Can you work these out from the drawing? Everything is in mm from the part's minimum corner. Give positions to 0.01 mm unless a question says otherwise; leave off trailing zeros. Loops run counter-clockwise (first coordinate to the right, second up) from the corner with the lowest first, then second, coordinate; pieces in that order, holes last. Notation, with made-up numbers: (1, -26) - (48, -26) arc R12 cw to (48, -6) - close; hole circle Ø8 at (23.25, 12). An arc over 180 degrees is marked (long way). Answer in a Markdown table with one row per item. Add a question column.
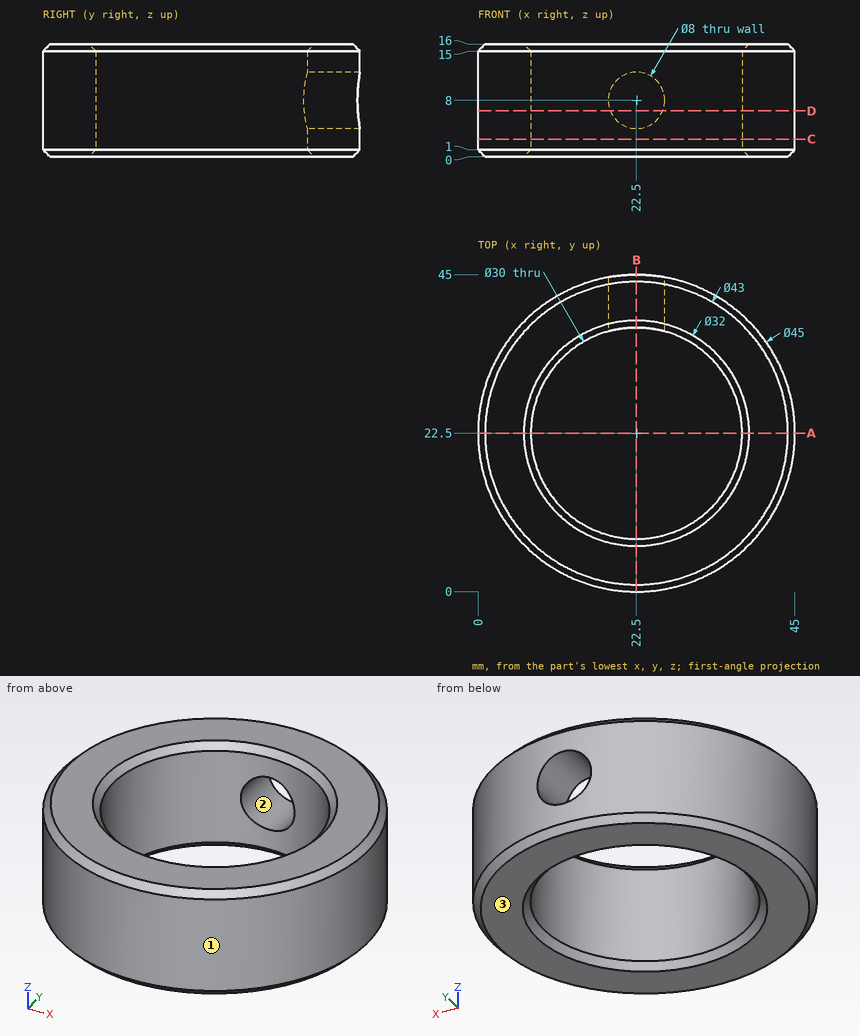
(1) For pin 1 Ø1 at (y, z) = (21, 1.5) entering from -X; pin 2 Ø3 at (x, z) = (31, 4) entering from +Y; pin 3 Ø8 at (y, z) = (31, 4) entering from +X, each with a flat end and sliding along its axis, tell me the tip position at first contact or that it passes through.
(2) I want a section at A-A on y = 22.5. Please give me the cut outline in (x, z).
(3) I want a section at D-D on z = 6.5. Please give me the cut outline in (x, y), then the cut area to 3 significant figures.
(4) We'd pull the mould along X, two halves only. Please class the marked faces 1, 2 and 3: pulls with the +X half, pulls with the -X half, needs draft (parallel to the pull), parting line crosses it, or undercut.
(5) I want a section at B-B on x = 22.5. Please give me the cut outline in (y, z), then the cut area to 3 significant figures.
(6) I want a section at C-C on z = 2.5. Please give me the cut outline in (x, y).
(7) Please list where these lines run through material, in increasing order: line 1 (Z direction, x = 22.5, y = 42); line 2 (Y direction, x = 22.5, z = 4.5); line 3 (X direction, y = 20, z = 2.25).
Reported:
| question | item | result |
|---|---|---|
| 1 | pin 1 | x = 0.02 |
| 1 | pin 2 | y = 43.88 |
| 1 | pin 3 | x = 44.55 |
| 2 | outline | (0, 1) - (1, 0) - (6.5, 0) - (7.5, 1) - (7.5, 15) - (6.5, 16) - (1, 16) - (0, 15) - close; (37.5, 1) - (38.5, 0) - (44, 0) - (45, 1) - (45, 15) - (44, 16) - (38.5, 16) - (37.5, 15) - close |
| 3 | outline | (18.79, 37.03) - (18.79, 44.69) arc R22.5 ccw (long way) to (26.21, 44.69) - (26.21, 37.03) arc R15 cw (long way) to start |
| 3 | area | 828 mm² |
| 4 | face 1 | parting line crosses it |
| 4 | face 2 | undercut |
| 4 | face 3 | needs draft |
| 5 | outline | (0, 1) - (1, 0) - (6.5, 0) - (7.5, 1) - (7.5, 15) - (6.5, 16) - (1, 16) - (0, 15) - close; (37.5, 1) - (38.5, 0) - (44, 0) - (45, 1) - (45, 4) - (37.5, 4) - close; (37.5, 12) - (45, 12) - (45, 15) - (44, 16) - (38.5, 16) - (37.5, 15) - close |
| 5 | area | 176 mm² |
| 6 | outline | circle Ø45 at (22.5, 22.5); hole circle Ø30 at (22.5, 22.5) |
| 7 | line 1 | 0 to 4, 12 to 16 |
| 7 | line 2 | 0 to 7.5 |
| 7 | line 3 | 0.14 to 7.71, 37.29 to 44.86 |
